Model file for the job. Use its own axes, mm. A direction names the side the tool comes from. Give positions to 0.01 mm unless a question says otherwise; leave off trailing zeros. Loops run counter-clockwise (first coordinate to the right, second up) from the corner with the lowest first, then second, coordinate; pieces in that order, holes last. Notation, with made-up numbers: (-16.5, -31) -> (-0.5, -31) arc R21 ccw to (-0.5, -11) -> close; hole circle Ø7 at (41.5, 36). An arc over 180 degrees is marked (long way). Use CSV: the item, a comma, the result in double quotes. Start each with the question number.
(1) Drill centre lines: probe 1 along X at (y, z) = (0.25, 77); probe 2 along Y at (x, z) = (0, 66.7). Where is each one in solid material? Low to high.
(2) Flat gauge pins, fed straight in: pin 1 (3 mm diameter, centred on y = -2.5, z = 24, fed in from +X); pin 2 (3 mm diameter, centred on x = 0, y = 0, fed in from +Z); pin 3 (1.5 mm diameter, centred on y = -7.5, z = 28.5, fed in from +X). Where does each tip first touch, or does it go through?
(3) Cut at B-B on x = 7. Write the cut outline in (y, z), then the cut area to 3 significant figures.
(4) 3-axis set-ups, long thin cutter, end or side, ignore diameter. For faces 1 (the flat face through (6, 1.647, 16)), 2 (the cylindrical face through (-1.437, 1.318, 80.14)), 3 (the flat face through (5, 2.647, 17)): which of +Z, -Z, +X, -X, +Y, -Y reach the whole face in a straight line?
(5) Pull direction X, two halves, no side cores. Call faces 4 (the cylindrical face through (-0.86, 0.27, 67.46)), 5 (the flat face through (1, -2, 0)), 6 (the flat face through (-2.647, -5, 17)): pulls with the +X half, pulls with the -X half, needs draft (parallel to the pull), parting line crosses it, or undercut.
(6) Cut at C-C on z = 37. Write the cut outline in (x, y).
(7) Cut at A-A on z = 24. Write the cut outline in (x, y), then the cut area to 3 significant figures.
from build123d import *

# Parameters (mm, degrees)
F0_R         = 2.95
F1_DEPTH     = 95
F3_DEPTH     = 35
F4_T4_DEPTH  = 1
F4_S5_R      = 2.95
F4_T6_DEPTH  = 8
F4_T10_DEPTH = 1
F4_S11_R     = 2.95
F4_T12_DEPTH = 8
F5_T4_DEPTH  = 37.2779404698
F5_T9_DEPTH  = 35.3377138687
F5_T14_DEPTH = 35.3377138687
F5_T19_DEPTH = 37.2779404698
F5_T21_DEPTH = 32
F9_R         = 1
F10_DEPTH    = 12.5
F11_DEPTH    = 5
F12_R        = 1.95
F13_DEPTH    = 20
F15_D        = 1.8
F15_DEPTH    = 5
F15_TIP      = 0.5407745571


# Not quite as in the source:
# - a fillet or chamfer that OpenCascade refuses, or shapes differently, is made with other operations: its cross-section is extruded or revolved along the edge and cut away or added


with BuildPart() as f1:
    # F0 (on Top) → F1 (new body)
    with BuildSketch(Plane.XY):
        Circle(F0_R)
    extrude(amount=F1_DEPTH)

    # F2 (on Top) → F3 (join)
    with BuildSketch(Plane.XY):
        Polygon((1.3030903237, 2.6465932079), (2.4476990844, 1.6465932079), (9.1030903237, 1.6465932079), (9.1030903237, 2.6465932079), align=None)
        Polygon((-2.6465932079, -9.1030903237), (-1.6465932079, -9.1030903237), (-1.6465932079, -2.4476990844), (-2.6465932079, -1.3030903237), align=None)
    extrude(amount=F3_DEPTH)

    # F4: chamfer of 8 on 2 edges, made by hand


with BuildPart() as f4_tool2:
    # F4_s3 → F4_t4 (new body)
    with BuildSketch(Plane.XZ.offset(-1.6465932079)):
        with BuildLine():
            Line((0.8768161537, 35.22627417), (9.3293644937, 26.77372583))
            Line((9.3293644937, 26.77372583), (9.4893644937, 26.77372583))
            ThreePointArc((9.4893644937, 26.77372583), (9.2630903237, 30.886862915), (9.2630903237, 35))
            Line((9.2630903237, 35), (9.1030903237, 35.16))
            ThreePointArc((9.1030903237, 35.16), (4.9899532387, 35.16), (0.8768161537, 35.38627417))
            Line((0.8768161537, 35.38627417), (0.8768161537, 35.22627417))
        make_face()
    extrude(amount=-F4_T4_DEPTH)

    # F4_s5 → F4_t6 (cut, symmetric)
    with BuildSketch(Plane.XY.offset(31.1)):
        Circle(F4_S5_R)
    extrude(amount=F4_T6_DEPTH, both=True, mode=Mode.SUBTRACT)


with BuildPart() as f1_1:
    add(f1.part)

    # F4_t1: cut F4_tool2
    add(f4_tool2.part, mode=Mode.SUBTRACT)


with BuildPart() as f4_tool8:
    # F4_s9 → F4_t10 (new body)
    with BuildSketch(Plane.YZ.offset(-2.6465932079)):
        with BuildLine():
            Line((-0.8768161537, 35.22627417), (-9.3293644937, 26.77372583))
            Line((-9.3293644937, 26.77372583), (-9.4893644937, 26.77372583))
            ThreePointArc((-9.4893644937, 26.77372583), (-9.2630903237, 30.886862915), (-9.2630903237, 35))
            Line((-9.2630903237, 35), (-9.1030903237, 35.16))
            ThreePointArc((-9.1030903237, 35.16), (-4.9899532387, 35.16), (-0.8768161537, 35.38627417))
            Line((-0.8768161537, 35.38627417), (-0.8768161537, 35.22627417))
        make_face()
    extrude(amount=F4_T10_DEPTH)

    # F4_s11 → F4_t12 (cut, symmetric)
    with BuildSketch(Plane.XY.offset(31.1)):
        Circle(F4_S11_R)
    extrude(amount=F4_T12_DEPTH, both=True, mode=Mode.SUBTRACT)


with BuildPart() as f1_2:
    add(f1_1.part)

    # F4_t7: cut F4_tool8
    add(f4_tool8.part, mode=Mode.SUBTRACT)

    # F5: fillet of radius 1 on 8 edges, made by hand


with BuildPart() as f5_tool2:
    # F5_s3 → F5_t4 (new body)
    with BuildSketch(Plane.XY):
        with BuildLine():
            ThreePointArc((-0.4828987249, -2.9102076939), (-1.2932405295, -3.1339296566), (-1.6465932079, -3.8967187765))
            Line((-1.6465932079, -3.8967187765), (-1.6465932079, -2.4476990844))
            ThreePointArc((-1.6465932079, -2.4476990844), (-1.0895698814, -2.7414115841), (-0.4828987249, -2.9102076939))
        make_face()
    extrude(amount=F5_T4_DEPTH)

    split(bisect_by=Plane(origin=(0, -18.0515451619, 18.0515451618), x_dir=(1, 0, 0), z_dir=(0, 0.7071067812, -0.7071067812)), keep=Keep.TOP)


with BuildPart() as f1_3:
    add(f1_2.part)

    # F5_t1: union F5_tool2
    add(f5_tool2.part)


with BuildPart() as f5_tool7:
    # F5_s8 → F5_t9 (new body)
    with BuildSketch(Plane.XY):
        with BuildLine():
            ThreePointArc((-2.723405054, -1.1338275494), (-2.6659841743, -1.3222015794), (-2.6465932079, -1.5181758712))
            Line((-2.6465932079, -1.5181758712), (-2.6465932079, -1.3030903237))
            ThreePointArc((-2.6465932079, -1.3030903237), (-2.6863325939, -1.2190640651), (-2.723405054, -1.1338275494))
        make_face()
    extrude(amount=F5_T9_DEPTH)

    split(bisect_by=Plane(origin=(0, -18.0515451619, 18.0515451618), x_dir=(1, 0, 0), z_dir=(0, 0.7071067812, -0.7071067812)), keep=Keep.TOP)


with BuildPart() as f1_4:
    add(f1_3.part)

    # F5_t6: union F5_tool7
    add(f5_tool7.part)


with BuildPart() as f5_tool12:
    # F5_s13 → F5_t14 (new body)
    with BuildSketch(Plane.XY):
        with BuildLine():
            ThreePointArc((1.1338275494, 2.723405054), (1.3222015794, 2.6659841743), (1.5181758712, 2.6465932079))
            Line((1.5181758712, 2.6465932079), (1.3030903237, 2.6465932079))
            ThreePointArc((1.3030903237, 2.6465932079), (1.2190640651, 2.6863325939), (1.1338275494, 2.723405054))
        make_face()
    extrude(amount=F5_T14_DEPTH)

    split(bisect_by=Plane(origin=(18.0515451619, 0, 18.0515451618), x_dir=(0, 1, 0), z_dir=(-0.7071067812, 0, -0.7071067812)), keep=Keep.TOP)


with BuildPart() as f1_5:
    add(f1_4.part)

    # F5_t11: union F5_tool12
    add(f5_tool12.part)


with BuildPart() as f5_tool17:
    # F5_s18 → F5_t19 (new body)
    with BuildSketch(Plane.XY):
        with BuildLine():
            ThreePointArc((2.9102076939, 0.4828987249), (3.1339296566, 1.2932405295), (3.8967187765, 1.6465932079))
            Line((3.8967187765, 1.6465932079), (2.4476990844, 1.6465932079))
            ThreePointArc((2.4476990844, 1.6465932079), (2.7414115841, 1.0895698814), (2.9102076939, 0.4828987249))
        make_face()
    extrude(amount=F5_T19_DEPTH)

    split(bisect_by=Plane(origin=(18.0515451619, 0, 18.0515451618), x_dir=(0, 1, 0), z_dir=(-0.7071067812, 0, -0.7071067812)), keep=Keep.TOP)


with BuildPart() as f1_6:
    add(f1_5.part)

    # F5_t16: union F5_tool17
    add(f5_tool17.part)

    # F5_s22 → F5_t21 (cut)
    with BuildSketch(Plane.XY.offset(-2.5)):
        with BuildLine():
            ThreePointArc((8.1030903237, 1.6465932079), (8.8101971049, 1.9394864268), (9.1030903237, 2.6465932079))
            Line((9.1030903237, 2.6465932079), (9.1030903237, 1.6465932079))
            Line((9.1030903237, 1.6465932079), (8.1030903237, 1.6465932079))
        make_face()
        with BuildLine():
            ThreePointArc((9.1030903237, 1.6465932079), (8.8101971049, 2.3536999891), (8.1030903237, 2.6465932079))
            Line((8.1030903237, 2.6465932079), (9.1030903237, 2.6465932079))
            Line((9.1030903237, 2.6465932079), (9.1030903237, 1.6465932079))
        make_face()
        with BuildLine():
            ThreePointArc((-2.6465932079, -8.1030903237), (-2.3536999891, -8.8101971049), (-1.6465932079, -9.1030903237))
            Line((-1.6465932079, -9.1030903237), (-2.6465932079, -9.1030903237))
            Line((-2.6465932079, -9.1030903237), (-2.6465932079, -8.1030903237))
        make_face()
        with BuildLine():
            ThreePointArc((-2.6465932079, -9.1030903237), (-1.9394864268, -8.8101971049), (-1.6465932079, -8.1030903237))
            Line((-1.6465932079, -8.1030903237), (-1.6465932079, -9.1030903237))
            Line((-1.6465932079, -9.1030903237), (-2.6465932079, -9.1030903237))
        make_face()
    extrude(amount=F5_T21_DEPTH, mode=Mode.SUBTRACT)

    # F9 (on 3pt) → F10 (cut, symmetric)
    with BuildSketch(Plane(origin=(0, 0, 0), x_dir=(0.7071067812, -0.7071067812, 0), z_dir=(-0.7071067812, -0.7071067812, 0))):
        Circle(F9_R)
    extrude(amount=F10_DEPTH, both=True, mode=Mode.SUBTRACT)

    # F11 (cut): a face of the model
    f11_faces = [f1_6.faces().sort_by_distance(p)[0] for p in [
        (0, 0, 95),
    ]]
    extrude(f11_faces, amount=-F11_DEPTH, mode=Mode.SUBTRACT)

    # F12 (on face) → F13 (cut)
    with BuildSketch(Plane.XY.offset(90)):
        Circle(F12_R)
    extrude(amount=-F13_DEPTH, mode=Mode.SUBTRACT)

    # F15
    with Locations(Plane.XY.offset(70)):
        with Locations((0, 0)):
            Hole(F15_D / 2, depth=F15_DEPTH)
            with Locations((0, 0, -(F15_DEPTH + F15_TIP / 2))):  # 118° drill point
                Cone(0, F15_D / 2, F15_TIP, mode=Mode.SUBTRACT)


solid = f1_6.part
Check result:
1,probe 1,"-2.94 to -1.93, 1.93 to 2.94"
1,probe 2,"-2.95 to -0.9, 0.9 to 2.95"
2,pin 1,"x = 2.78"
2,pin 2,"z = 70"
2,pin 3,"x = -1.65"
3,outline,"(1.65, 0) -> (2.65, 0) -> (2.65, 29.1) -> (1.65, 29.1) -> close"
3,area,"29.1 mm²"
4,face 1,"+Z, -Z, +X, -Y"
4,face 2,"+Z"
4,face 3,"+Z, -Z, +X, +Y"
5,face 4,"undercut"
5,face 5,"needs draft"
5,face 6,"pulls with the -X half"
6,outline,"circle Ø5.9 at (0, 0)"
7,outline,"(-2.72, -1.13) arc R1 cw to (-2.65, -1.52) -> (-2.65, -8.1) arc R1 ccw to (-2.15, -8.97) arc R1 ccw to (-1.65, -8.1) -> (-1.65, -3.9) arc R1 cw to (-0.48, -2.91) arc R2.95 ccw to (2.91, 0.48) arc R1 cw to (3.9, 1.65) -> (8.1, 1.65) arc R1 ccw to (8.97, 2.15) arc R1 ccw to (8.1, 2.65) -> (1.52, 2.65) arc R1 cw to (1.13, 2.72) arc R2.95 ccw to start"
7,area,"41.7 mm²"
